Here's how the part is built. I have some questions about the finished solid (model axes, mm). Round coordinates to 2 decimals unless told otherwise and drop trailing zeros. Loops run counter-clockwise (first coordinate to the right, second up) from the corner with the lowest first, then second, coordinate; pieces in that order, holes last. Notation, with made-up numbers: M -5,89.5 L 16,89.5 A25 ccw 16,119.5 Z; hole C 61,39.25 d10. An arc over 180 degrees is marked long. Use a Markdown table: item, result.
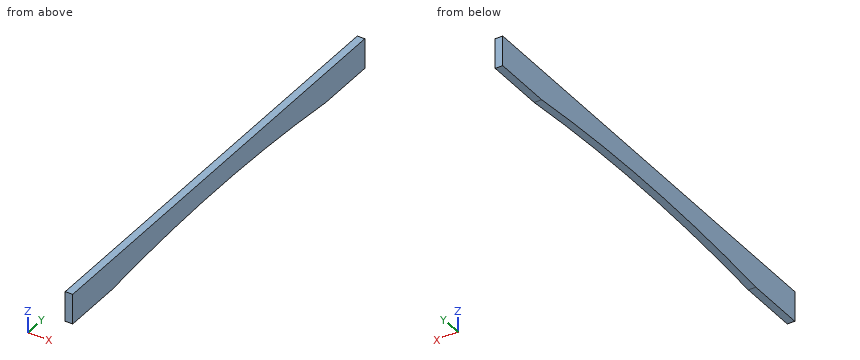
```python
from build123d import *

# Parameters (mm, degrees)
F1_DEPTH = 25.4


with BuildPart() as f1:
    # F0 (on Right) → F1 (new body)
    with BuildSketch(Plane.YZ):
        with BuildLine():
            Line((762, 64.476146), (-762, 64.476146))
            Line((-762, 64.476146), (-762, -37.123854))
            Line((-762, -37.123854), (-558.8, -37.123854))
            ThreePointArc((-558.8, -37.123854), (0, -7.803793), (558.8, -37.123854))
            Line((558.8, -37.123854), (762, -37.123854))
            Line((762, -37.123854), (762, 64.476146))
        make_face()
    extrude(amount=-F1_DEPTH)


solid = f1.part
```
Q1. Imagine slicing it at B-B, the plane x = -14. Please give me the cut outline in (y, z), then the cut area to 3 significant figures.
Return value:
| item | result |
|---|---|
| outline | M -762,-37.12 L -558.8,-37.12 A5339.64 cw 558.8,-37.12 L 762,-37.12 L 762,64.48 L -762,64.48 Z |
| area | 133,000 mm^2 |
Q2. Imagine slicing it at C-C, the plane y = -121. Please give me the cut outline in (x, z).
Return value:
| item | result |
|---|---|
| outline | M -25.4,-9.17 L 0,-9.17 L 0,64.48 L -25.4,64.48 Z |
Q3. Will this pin go through, and if not, where does the flat tip stop? P1, Ø12, axis at y = 510, z = 0.5, coming from the +X side.
Return value:
| item | result |
|---|---|
| P1 | stops at x = 0 |
Q4. Imagine slicing it at D-D, the plane y = -449. Please give me the cut outline in (x, z).
Return value:
| item | result |
|---|---|
| outline | M -25.4,-26.72 L 0,-26.72 L 0,64.48 L -25.4,64.48 Z |
Q5. Imagine slicing it at A-A, the plane z = -24.5. Please give me the cut outline in (x, y), then the cut area to 3 significant figures.
Return value:
| item | result |
|---|---|
| outline | M -25.4,-762 L 0,-762 L 0,-421.93 L -25.4,-421.93 Z; M -25.4,421.93 L 0,421.93 L 0,762 L -25.4,762 Z |
| area | 17,300 mm^2 |
Q6. I need wall thicknesses on line 1 (Z direction, x = -19.25, y = -22.5); line 2 (Z direction, x = -4.75, y = -380.5). Which ranges of each line are inside material? Lowest first, please. Write a range as from..to.
Return value:
| item | result |
|---|---|
| line 1 | z = -7.85..64.48 |
| line 2 | z = -21.38..64.48 |
